from build123d import *

# Parameters (mm, degrees)
SKETCH1_R                       = 14.2875
BOSS_EXTRUDE1_DEPTH             = 6.35
F_10_CLEARANCE_HOLE1_AT_2_COUNT = 2
F_10_CLEARANCE_HOLE1_AT_2_PITCH = 38.625542067
F_10_CLEARANCE_HOLE1_AT_3_COUNT = 2
F_10_CLEARANCE_HOLE1_AT_3_PITCH = 61.237182332
F_10_CLEARANCE_HOLE1_AT_4_COUNT = 2
F_10_CLEARANCE_HOLE1_AT_4_PITCH = 82.55


with BuildPart() as part:
    # Sketch1 → Boss-Extrude1 (new body)
    with BuildSketch(Plane(origin=(0, 0, 0), x_dir=(1, 0, 0), z_dir=(0, 1, 0))):
        with BuildLine():
            Line((-16.703230912, 5.093229167), (-6.07390215, 39.952083333))
            ThreePointArc((-6.07390215, 39.952083333), (0, 44.45), (6.07390215, 39.952083333))
            Line((6.07390215, 39.952083333), (12.644794548, 18.402859955))
            Line((12.644794548, 18.402859955), (21.547953627, 19.034099518))
            ThreePointArc((21.547953627, 19.034099518), (27.49630657, 15.875), (27.257990535, 9.144025482))
            Line((27.257990535, 9.144025482), (21.077367113, 0))
            Line((21.077367113, 0), (27.257990535, -9.144025482))
            ThreePointArc((27.257990535, -9.144025482), (27.49630657, -15.875), (21.547953627, -19.034099518))
            Line((21.547953627, -19.034099518), (13.272110504, -18.44733705))
            Line((13.272110504, -18.44733705), (6.148361062, -46.0375))
            ThreePointArc((6.148361062, -46.0375), (0, -50.8), (-6.148361062, -46.0375))
            Line((-6.148361062, -46.0375), (-16.907992921, -4.365625))
            ThreePointArc((-16.907992921, -4.365625), (-17.458409791, 0.377933626), (-16.703230912, 5.093229167))
        make_face()
        with Locations(Location((0, 0, 0), (0, 0, 270))):
            Circle(SKETCH1_R, mode=Mode.SUBTRACT)
    extrude(amount=BOSS_EXTRUDE1_DEPTH)

    # Sketch3 → #10 Clearance Hole1 (revolve, cut)
    with BuildSketch(Plane(origin=(0, 6.35, 44.45), x_dir=(0, 0, 1), z_dir=(1, 0, 0))):
        Polygon((0, 0), (0, 6.35), (3.1877, 6.35), (2.5527, 5.715), (2.5527, 0.635), (3.1877, 0), align=None)
    f_10_clearance_hole1 = revolve(axis=Axis((0, 12.7, 44.45), (0, -1, 0)), mode=Mode.SUBTRACT)

    # #10 Clearance Hole1 at 2: #10 Clearance Hole1 ×2
    with Locations(*[Vector(0.5694947974514997, 0, -0.8219949365267863) * (i * F_10_CLEARANCE_HOLE1_AT_2_PITCH) for i in range(1, F_10_CLEARANCE_HOLE1_AT_2_COUNT)]):
        add(f_10_clearance_hole1, mode=Mode.SUBTRACT)

    # #10 Clearance Hole1 at 3: #10 Clearance Hole1 ×2
    with Locations(*[Vector(0.3592106040535505, 0, -0.9332565252573826) * (i * F_10_CLEARANCE_HOLE1_AT_3_PITCH) for i in range(1, F_10_CLEARANCE_HOLE1_AT_3_COUNT)]):
        add(f_10_clearance_hole1, mode=Mode.SUBTRACT)

    # #10 Clearance Hole1 at 4: #10 Clearance Hole1 ×2
    with Locations(*[(0, 0, -i * F_10_CLEARANCE_HOLE1_AT_4_PITCH) for i in range(1, F_10_CLEARANCE_HOLE1_AT_4_COUNT)]):
        add(f_10_clearance_hole1, mode=Mode.SUBTRACT)


solid = part.part
Read the model definition and answer for the solid it produces. Units are mm, in the model's axes. A direction names the side the tool comes from. Give positions to 0.01 mm unless a question says otherwise; leave off trailing zeros. Write each loop counter-clockwise with the first axis right and the second up, starting at its lowest first coordinate (ties: lowest second). Pieces come first, ordered by that corner, then holes. Notation, with made-up numbers: (61.5, -31.75) - (89.5, -31.75) arc R11 cw to (89.5, -25.75) - close; hole circle Ø2 at (65.5, -37.75). An arc over 180 degrees is marked (long way). Use CSV: the item, a comma, the result in double quotes. Start each with the question number.
(1) For faces 1 (the flat face through (24.211, 3.131, -4.636)), 2 (the cylindrical face through (-0.1, 3.2, 41.9)), 3 (the flat face through (17.468, 3.131, 18.745)), determine the directions among +Z, -Z, +X, -X, +Y, -Y from which every point of the face is accessible in a straight line to the end or side of a thin tool.
(2) Consider line 1 along Z through (x, y) = (20, 2.25); line 2 along Z through (x, y) = (20.5, 5); line 3 along X through (y, z) = (2.6, 12.7). Determine where each line is inside the solid, lowest interval first.
(3) Given P1, Ø23, axis at x = 0, z = 0, coming from the -Y side; P2, Ø1.5, axis at y = 5.5, z = 29, coming from the -X side; P3, Ø1, axis at x = -3.5, y = 2, coming from the +Z side, each flat-ended and moving along its own axis, determine where each tip first touches the part or whether it passes through.
(4) Find section A-A (x = 0). Count the separate pieces of the cut face and the enclosed holes in it, plus the area to 3 significant figures.
(5) Find section B-B (z = -38.1). Give the vertices of the cut face in (x, y) (3 decimals).
(6) Find section D-D (z = 44.45). Give the vertices of the cut face in (x, y) (3 decimals).
(7) Determine the mould class of faces 4 (the flat face through (24.124, 3.131, 4.508)), 5 (the flat face through (17.034, 3.131, -18.714)), 6 (the cylindrical face through (-17.46, 3.13, -0.31)) for opening direction X: +X half, -X half, draft (parallel to the pull), parting line (faces both ways), or undercut.
Findings below:
1,face 1,"+X, +Y, -Y"
1,face 2,"+Y, -Y"
1,face 3,"+Z, +Y, -Y"
2,line 1,"-18.92 to -14.29, -11.11 to 11.11, 14.29 to 18.92"
2,line 2,"-18.96 to -14.77, -10.63 to 10.63, 14.77 to 18.96"
2,line 3,"-14.76 to -6.55, 6.55 to 19.44, 24.55 to 28.35"
3,P1,"through"
3,P2,"x = -10.74"
3,P3,"z = 50.05"
4,separate pieces,"4"
4,enclosed holes,"0"
4,area,"357 mm2"
5,outline,"(-6.639, 0) - (-3.188, 0) - (-2.553, 0.635) - (-2.553, 5.715) - (-3.188, 6.35) - (-6.639, 6.35) - close; (2.553, 0.635) - (3.188, 0) - (6.639, 0) - (6.639, 6.35) - (3.188, 6.35) - (2.553, 5.715) - close"
6,outline,"(-6.558, 0) - (-3.188, 0) - (-2.553, 0.635) - (-2.553, 5.715) - (-3.188, 6.35) - (-6.558, 6.35) - close; (2.553, 0.635) - (3.188, 0) - (6.558, 0) - (6.558, 6.35) - (3.188, 6.35) - (2.553, 5.715) - close"
7,face 4,"+X half"
7,face 5,"undercut"
7,face 6,"-X half"
